```python
from build123d import *

# Parameters (mm, degrees)
F1_DEPTH = 6.35
F2_W     = 3.81
F2_H     = 3.81
F3_DEPTH = 3.81


with BuildPart() as f1:
    # F0 (on Front) → F1 (new body)
    with BuildSketch(Plane.XZ):
        with BuildLine():
            ThreePointArc((-50.8, -12.7), (-48.940128, -17.190128), (-44.45, -19.05))
            Line((-44.45, -19.05), (44.45, -19.05))
            ThreePointArc((44.45, -19.05), (48.940128, -17.190128), (50.8, -12.7))
            Line((50.8, -12.7), (50.8, 12.7))
            ThreePointArc((50.8, 12.7), (48.940128, 17.190128), (44.45, 19.05))
            Line((44.45, 19.05), (-44.45, 19.05))
            ThreePointArc((-44.45, 19.05), (-48.940128, 17.190128), (-50.8, 12.7))
            Line((-50.8, 12.7), (-50.8, -12.7))
        make_face()
    extrude(amount=F1_DEPTH)

    # F2 (on face) → F3 (join)
    with BuildSketch(Plane.XZ.offset(6.35)):
        with Locations((-39.331302, 0)):
            Rectangle(F2_W, F2_H)
    extrude(amount=F3_DEPTH)


solid = f1.part
```
The model under review builds one solid part; all positions refer to its coordinate system, in mm. A direction names the side the tool comes from. Round coordinates to 2 decimals unless told otherwise and drop trailing zeros. Write each loop counter-clockwise with the first axis right and the second up, starting at its lowest first coordinate (ties: lowest second). Pieces come first, ordered by that corner, then holes. Notation, with made-up numbers: (57.5, 59.25) -> (107.5, 59.25) arc R16 cw to (107.5, 81.25) -> close; hole circle Ø5 at (31.5, 58.25). An arc over 180 degrees is marked (long way). Use CSV: the item, a comma, the result in double quotes.
Q1. To check wall thickness, follow probe 1 along Y at (x, z) = (-10.5, 4.5); probe 2 along X at (y, z) = (-5, -13); probe 3 along Z at (x, y) = (-39, -9.5) (3 decimals). State the ranges of each line that lie inside material, in increasing order. Write a range as [from, to].
Checks:
probe 1,"[-6.35, 0]"
probe 2,"[-50.79, 50.79]"
probe 3,"[-1.905, 1.905]"
Q2. Consider section B-B (y = -7.75). Give the boundary of the cut face in (x, z) (3 decimals).
Checks:
outline,"(-41.236, -1.905) -> (-37.426, -1.905) -> (-37.426, 1.905) -> (-41.236, 1.905) -> close"
Q3. For pin 1 Ø3 at (x, y) = (-40, -8) entering from -Z (3 decimals); pin 2 Ø1.1 at (y, z) = (-7.5, 0.5) entering from -X; pin 3 Ø1.9 at (y, z) = (-8.5, 1) entering from +X, all flat-tipped, find the tip position at first contact; note any pin that passes through.
Checks:
pin 1,"z = -1.905"
pin 2,"x = -41.24"
pin 3,"x = -37.43"
Q4. Consider section A-A (z = 0). Give the boundary of the cut face in (x, y), then the cut area to 3 significant figures.
Checks:
outline,"(-50.8, -6.35) -> (-41.24, -6.35) -> (-41.24, -10.16) -> (-37.43, -10.16) -> (-37.43, -6.35) -> (50.8, -6.35) -> (50.8, 0) -> (-50.8, 0) -> close"
area,"660 mm²"
Q5. Consider section C-C (x = 27). Give the boundary of the cut face in (y, z), then the cut area to 3 significant figures.
Checks:
outline,"(-6.35, -19.05) -> (0, -19.05) -> (0, 19.05) -> (-6.35, 19.05) -> close"
area,"242 mm²"
Q6. For faces 1 (the flat face through (-39, -8, -1.905)), 2 (the cylindrical face through (-48.99, -3.13, -17.14)), 3 (the flat face through (-41.236, -8, 0)), 4 (the flat face through (-39, -8, 1.905)), 5 (the flat face through (-37.426, -8, 0)), list the 3-axis set-ups (+Z, -Z, +X, -X, +Y, -Y) from which the entire face can be reached by the end or side of a thin tool; tool diameter is ignored.
Checks:
face 1,"-Z, +X, -X, -Y"
face 2,"-Z, -X, +Y, -Y"
face 3,"+Z, -Z, -X, -Y"
face 4,"+Z, +X, -X, -Y"
face 5,"+Z, -Z, +X, -Y"
